from build123d import *

# Parameters (mm, degrees)
BOSS_EXTRUDE1_DEPTH = 6.35


with BuildPart() as part:
    # Sketch1 → Boss-Extrude1 (new body)
    with BuildSketch(Plane(origin=(0, 0, 0), x_dir=(1, 0, 0), z_dir=(0, 1, 0))):
        with BuildLine():
            Line((-115, -64.215517859), (-105, -64.215517859))
            Line((-105, -64.215517859), (-105, 23.784482141))
            Line((-105, 23.784482141), (-70, 23.784482141))
            Line((-70, 23.784482141), (-70, 33.784482141))
            Line((-70, 33.784482141), (-19, 33.784482141))
            Line((-19, 33.784482141), (-19, 48.284482141))
            Line((-19, 48.284482141), (46.5, 48.284482141))
            Line((46.5, 48.284482141), (46.5, 9.784482141))
            Line((46.5, 9.784482141), (74.5, 9.784482141))
            Line((74.5, 9.784482141), (74.5, 7.284482141))
            add(Edge.make_bspline(
                [(74.5, 7.284482141), (78.941812559, 8.679963078), (89.598105333, 14.160361523), (96.061867219, 23.189471951), (96.610613644, 29.034482141)],
                knots=[0, 0, 0, 0, 0.139776101, 0.343963844, 0.343963844, 0.343963844, 0.343963844], degree=3))
            Line((96.610613644, 29.034482141), (101.594478802, 29.034482141))
            add(Edge.make_bspline(
                [(75.956941241, 2.501457761), (80.440075067, 3.907014197), (86.917003439, 7.092067173), (94.089056782, 13.146274012), (98.414454942, 18.57956616), (100.864778933, 24.020415983), (101.497230208, 27.680092848), (101.594478802, 29.034482141)],
                knots=[0, 0, 0, 0, 0.125, 0.1875, 0.25, 0.3125, 0.348130447, 0.348130447, 0.348130447, 0.348130447], degree=3))
            Line((75.956941241, 2.501457761), (74.5, 2.284482141))
            Line((74.5, 2.284482141), (74.5, -0.215517859))
            Line((74.5, -0.215517859), (46.5, -0.215517859))
            Line((46.5, -0.215517859), (46.5, -17.215517859))
            Line((46.5, -17.215517859), (-19, -17.215517859))
            Line((-19, -17.215517859), (-19, -2.215517859))
            Line((-19, -2.215517859), (-28, -2.215517859))
            Line((-28, -2.215517859), (-28, 12.784482141))
            Line((-28, 12.784482141), (-95, 12.784482141))
            Line((-95, 12.784482141), (-95, -64.215517859))
            Line((-95, -64.215517859), (115, -64.215517859))
            Line((115, -64.215517859), (115, 64.215517859))
            Line((115, 64.215517859), (-115, 64.215517859))
            Line((-115, 64.215517859), (-115, -64.215517859))
        make_face()
    extrude(amount=BOSS_EXTRUDE1_DEPTH)


solid = part.part
Source: CAD feature listing. Evaluate the final solid. Frame: model axes, mm. A direction names the side the tool comes from. Coordinates: 2 decimals unless noted, no trailing zeros. Loops run counter-clockwise (first coordinate to the right, second up) from the corner with the lowest first, then second, coordinate; pieces in that order, holes last. Notation, with made-up numbers: (79.25, -18) -> (95.25, -18) arc R14 cw to (95.25, 0) -> close; hole circle Ø10 at (59.25, -9). An arc over 180 degrees is marked (long way). Answer in a Markdown table with one row per item. Add a question column.
Q1. Section B-B on x = -25. Return the cut outline in (y, z).
Q2. Reachability of faces 1 (the face through (-105, 3, 21)), 2 (the face through (-88, 3, -23.784)) from +Z, -Z, +X, -X, +Y, -Y: full face, straight path, thin tool, end or side. Return the list, or none.
Q3. Ray query, line 1 along X through (y, z) = (5, 0.5); line 2 along X through (y, z) = (3, 7); line 3 along Z through (x, y) = (-74.5, 5.5). Return the intervals inside material, ascending.
Q4. Section C-C on z = 13. Return the cut outline in (x, y).
Q5. Pull-direction query (X, two-part tool) for faces 3 (the face through (-70, 3, -29)), 4 (the face through (-45, 3, -33.784)), 5 (the face through (-110, 3, 64.216)), 6 (the face through (-115, 3, -1)); classes: pulls with the +X half, pulls with the -X half, needs draft (parallel to the pull), parting line crosses it, or undercut.
Q6. Section A-A on z = -42.5. Return the cut outline in (x, y), and give its area (3 significant figures).
Computed values:
| question | item | result |
|---|---|---|
| 1 | outline | (0, -64.22) -> (6.35, -64.22) -> (6.35, -33.78) -> (0, -33.78) -> close; (0, 2.22) -> (6.35, 2.22) -> (6.35, 64.22) -> (0, 64.22) -> close |
| 2 | face 1 | +Z, +Y, -Y |
| 2 | face 2 | +Y, -Y |
| 3 | line 1 | x = -115 to -105, -95 to -28, 46.5 to 115 |
| 3 | line 2 | x = -115 to -105, -95 to -19, 46.5 to 115 |
| 3 | line 3 | z = -64.22 to -23.78, -12.78 to 64.22 |
| 4 | outline | (-115, 0) -> (-105, 0) -> (-105, 6.35) -> (-115, 6.35) -> close; (-95, 0) -> (-19, 0) -> (-19, 6.35) -> (-95, 6.35) -> close; (46.5, 0) -> (115, 0) -> (115, 6.35) -> (46.5, 6.35) -> close |
| 5 | face 3 | undercut |
| 5 | face 4 | undercut |
| 5 | face 5 | needs draft |
| 5 | face 6 | pulls with the -X half |
| 6 | outline | (-115, 0) -> (-19, 0) -> (-19, 6.35) -> (-115, 6.35) -> close; (46.5, 0) -> (115, 0) -> (115, 6.35) -> (46.5, 6.35) -> close |
| 6 | area | 1,040 mm^2 |
